For this review, take the finished solid that the model builds, in its own axes (mm). Face numbers are marked on the shaded views. A direction names the side the tool comes from. Coordinates: 2 decimals unless noted, no trailing zeros. Write each loop counter-clockwise with the first axis right and the second up, starting at its lowest first coordinate (ties: lowest second). Pieces come first, ordered by that corner, then holes.
1) For the marked faces 4, 5 and 6, list the 3-axis set-ups (+Z, -Z, +X, -X, +Y, -Y) from which the entire face can be reached by the end or side of a thin tool; tool diameter is ignored.
2) We need section A-A on x = 0. Write out the cut boundary in (y, z), then the cut area to 3 significant figures.
3) Insertion check: P1, Ø5, axis at x = -5.5, y = 49.5, coming from the -Z side; P2, Ø3, axis at x = -22.5, y = 27, coming from the -Z side; P3, Ø1, axis at x = -13, y = 15.5, coming from the -Z side. Each pin has a flat end and moves straight along its axis. Give the tip position at first contact, or say it passes through.
4) We need section B-B on z = 0. Write out the cut boundary in (x, y), then the cut area to 3 significant figures.
5) We need section C-C on y = 67.5. Write out the cut boundary in (x, z).
6) Mouldability with a two-part tool opening along Z and no side actions: class the marked faces 1, 2 and 3 as pulls with the +Z half, pulls with the -Z half, needs draft (parallel to the pull), parting line crosses it, or undercut.
7) We need section D-D on x = -25.5. Write out the cut boundary in (y, z).
8) To check wall thickness, follow line 1 along Y through (x, z) = (-30, -1.5); line 2 along X through (y, z) = (56, 0); line 3 along X through (y, z) = (18, 0). State the ranges of each line that lie inside material, in increasing order.
from build123d import *

# Parameters (mm, degrees)
SKETCH3_R          = 1.5
CUT_EXTRUDE1_DEPTH = 5


with BuildPart() as part:
    # Sketch2 → Revolve1 (revolve)
    with BuildSketch(Plane.XY, mode=Mode.PRIVATE) as revolve1_sk:
        Polygon((-22, 0), (-31, 0), (-31, 10), (-29.5, 10), (-29.5, 47), (-31, 47), (-31, 58), (-38, 58), (-38, 69), (-41.5, 69), (-41.5, 77), (-22, 77), align=None)
    revolve(revolve1_sk.sketch.rotate(Axis((0, 108.342465753, 0), (0, -1, 0)), 270), axis=Axis((0, 108.342465753, 0), (0, -1, 0)))  # turned: the seam where the file's is

    # Sketch3 → Cut-Extrude1 (cut)
    with BuildSketch(Plane.XZ):
        with Locations((-22, 0)):
            Circle(SKETCH3_R)
    extrude(amount=-CUT_EXTRUDE1_DEPTH, mode=Mode.SUBTRACT)


solid = part.part
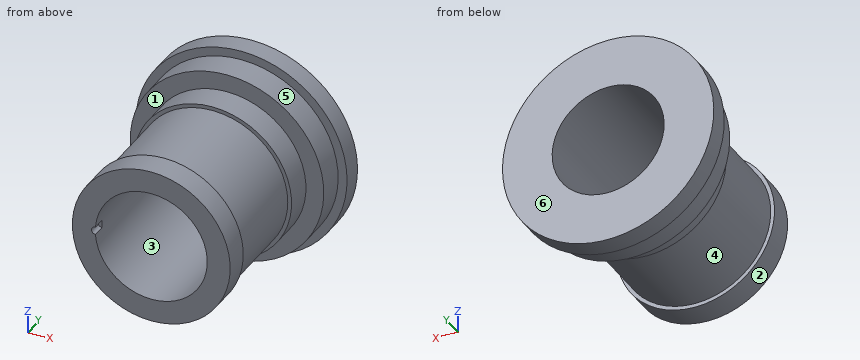
Result:
1. face 4: none
1. face 5: -Y
1. face 6: +Z, -Z, +X, -X, +Y
2. outline: (0, -31) - (10, -31) - (10, -29.5) - (47, -29.5) - (47, -31) - (58, -31) - (58, -38) - (69, -38) - (69, -41.5) - (77, -41.5) - (77, -22) - (0, -22) - close; (0, 22) - (77, 22) - (77, 41.5) - (69, 41.5) - (69, 38) - (58, 38) - (58, 31) - (47, 31) - (47, 29.5) - (10, 29.5) - (10, 31) - (0, 31) - close
2. area: 1,600 mm2
3. P1: stops at z = -30.85
3. P2: stops at z = -20.72
3. P3: stops at z = -26.72
4. outline: (-41.5, 69) - (-38, 69) - (-38, 58) - (-31, 58) - (-31, 47) - (-29.5, 47) - (-29.5, 10) - (-31, 10) - (-31, 0) - (-23.5, 0) - (-23.5, 5) - (-22, 5) - (-22, 77) - (-41.5, 77) - close; (22, 0) - (31, 0) - (31, 10) - (29.5, 10) - (29.5, 47) - (31, 47) - (31, 58) - (38, 58) - (38, 69) - (41.5, 69) - (41.5, 77) - (22, 77) - close
4. area: 1,590 mm2
5. outline: circle Ø76 at (0, 0); hole circle Ø44 at (0, 0)
6. face 1: needs draft
6. face 2: parting line crosses it
6. face 3: undercut
7. outline: (0, -17.63) - (10, -17.63) - (10, -14.83) - (47, -14.83) - (47, -17.63) - (58, -17.63) - (58, -28.17) - (69, -28.17) - (69, -32.74) - (77, -32.74) - (77, 32.74) - (69, 32.74) - (69, 28.17) - (58, 28.17) - (58, 17.63) - (47, 17.63) - (47, 14.83) - (10, 14.83) - (10, 17.63) - (0, 17.63) - close
8. line 1: y = 0 to 10, 47 to 77
8. line 2: x = -31 to -22, 22 to 31
8. line 3: x = -29.5 to -22, 22 to 29.5
